from build123d import *

# Parameters (mm, degrees)
SKETCH_1_W          = 10
SKETCH_1_H          = 12
SKETCH_1_R          = 3.5
EXTRUDE_1_DEPTH     = 1.7
SKETCH_2_R          = 0.7
CUT_EXTRUDE_1_DEPTH = 8.993122043
CUT_EXTRUDE_START   = -1.7
SKETCH_2_3_R        = 1
CUT_EXTRUDE_2_DEPTH = 1


with BuildPart() as part:
    # 草图1 → 凸台-拉伸1 (new body)
    with BuildSketch(Plane(origin=(0, 0, 0), x_dir=(1, 0, 0), z_dir=(0, 1, 0))):
        Rectangle(SKETCH_1_W, SKETCH_1_H)
        with Locations(Location((0, 0, 0), (0, 0, 270))):
            Circle(SKETCH_1_R, mode=Mode.SUBTRACT)
    extrude(amount=EXTRUDE_1_DEPTH)

    # 草图2 → 切除-拉伸1 (cut, through all)
    with BuildSketch(Plane.XZ):
        with Locations(Location((0, 5.05, 0), (0, 0, 270))):
            Circle(SKETCH_2_R)
        with Locations(Location((3.5, -4.5, 0), (0, 0, 270))):
            Circle(SKETCH_2_R)
        with Locations(Location((-3.5, -4.5, 0), (0, 0, 270))):
            Circle(SKETCH_2_R)
    extrude(amount=-CUT_EXTRUDE_1_DEPTH, mode=Mode.SUBTRACT)

    # 草图2<3> → 切除-拉伸2 (cut)
    with BuildSketch(Plane.XZ.offset(CUT_EXTRUDE_START)):
        with Locations((0, 5.05)):
            Circle(SKETCH_2_3_R)
        with Locations(Location((3.5, -4.5, 0), (0, 0, 270))):
            Circle(SKETCH_2_3_R)
        with Locations(Location((-3.5, -4.5, 0), (0, 0, 270))):
            Circle(SKETCH_2_3_R)
    extrude(amount=CUT_EXTRUDE_2_DEPTH, mode=Mode.SUBTRACT)


solid = part.part
Verification items for the finished model (mm, model axes). A direction names the side the tool comes from. Coordinates: 2 decimals unless noted, no trailing zeros. Order: outer loops, then holes, each group sorted by start corner. A loop starts at its lowest first (then second) coordinate and runs counter-clockwise, first axis right, second up. Notation, with made-up numbers: M 23,-17 L 77,-17 A37 ccw 77,20 Z; hole C -10,8.5 d10. An arc over 180 degrees is marked long. One line per item, written item: value. Start each with the question number.
Item 1: Access from +Z, -Z, +X, -X, +Y, -Y to the whole of each face (thin tool, end or side, straight path). Record for faces 4 (the cylindrical face through (4.176, 1.207, -3.763)), 5 (the cylindrical face through (0.03, 0.35, 5.75)).
Item 2: Sectioned sample at A-A on z = 5.05. Record the cut outline in (x, y).
Item 3: Mould release check, pull along X, two halves, no side actions. Record for faces 1 (the flat face through (-5, 1, 0)), 2 (the cylindrical face through (-0.04, 1.21, 4.05)), 3 (the flat face through (-3.4, 0, -1.4)): pulls with the +X half, pulls with the -X half, needs draft (parallel to the pull), parting line crosses it, or undercut.
Item 4: Sectioned sample at B-B on x = -1.75. Record the cut outline in (y, z), then the cut area to 3 significant figures.
Item 5: Sectioned sample at D-D on y = 1.5. Record the cut outline in (x, z), then the cut area to 3 significant figures.
Item 6: Thickness scan on probe 1 along X at (y, z) = (0.95, -4.5); probe 2 along X at (y, z) = (0.3, 5.05); probe 3 along Z at (x, y) = (3, 0.2). Record the ranges inside material, lowest first.
Item 7: Sectioned sample at C-C on z = -4.5. Record the cut outline in (x, y).
Item 8: Depth check by flat-ended pin: P1, Ø0.6, axis at x = -0.5, z = 5, coming from the +Y side. Enter the tip coordinate at first touch or a pass-through.
Calculated:
1. face 4: +Y
1. face 5: +Y, -Y
2. outline: M -5,0 L -0.7,0 L -0.7,0.7 L -1,0.7 L -1,1.7 L -5,1.7 Z; M 0.7,0 L 5,0 L 5,1.7 L 1,1.7 L 1,0.7 L 0.7,0.7 Z
3. face 1: pulls with the -X half
3. face 2: undercut
3. face 3: needs draft
4. outline: M 0,-6 L 1.7,-6 L 1.7,-3.03 L 0,-3.03 Z; M 0,3.03 L 1.7,3.03 L 1.7,6 L 0,6 Z
4. area: 10.1 mm^2
5. outline: M -5,-6 L 5,-6 L 5,6 L 0.31,6 A1 cw long -0.31,6 L -5,6 Z; hole C -3.5,-4.5 d2; hole C 0,0 d7; hole C 3.5,-4.5 d2
5. area: 72.1 mm^2
6. probe 1: -5 to -4.5, -2.5 to 2.5, 4.5 to 5
6. probe 2: -5 to -0.7, 0.7 to 5
6. probe 3: -6 to -4.99, -4.01 to -1.8, 1.8 to 6
7. outline: M -5,0 L -4.2,0 L -4.2,0.7 L -4.5,0.7 L -4.5,1.7 L -5,1.7 Z; M -2.8,0 L 2.8,0 L 2.8,0.7 L 2.5,0.7 L 2.5,1.7 L -2.5,1.7 L -2.5,0.7 L -2.8,0.7 Z; M 4.2,0 L 5,0 L 5,1.7 L 4.5,1.7 L 4.5,0.7 L 4.2,0.7 Z
8. P1: y = 0.7
